Verification items for the finished model (mm, model axes). A direction names the side the tool comes from. Round coordinates to 2 decimals unless told otherwise and drop trailing zeros. Write each loop counter-clockwise with the first axis right and the second up, starting at its lowest first coordinate (ties: lowest second). Pieces come first, ordered by that corner, then holes. Notation, with made-up numbers: (31, 43) - (74, 43) arc R16 ccw to (74, 58) - close; hole circle Ø8 at (6, 34). An arc over 180 degrees is marked (long way). Answer as a JSON object with one key per item and string values. Group by question number.
1) Section check B-B (y = -5.5). Enter the section's corners in (x, z).
2) Mould release check, pull along Z, two halves, no side actions. Record for faces 4 (the flat face through (165, 13, 7)), 5 (the flat face through (74, 13, 0)), 6 (the cylindrical face through (31.952, -14.132, 7.934)): +Z half, -Z half, draft (parallel to the pull), parting line (faces both ways), or undercut.
3) Section check C-C (y = 21.5). Enter the section's corners in (x, z).
4) Go/stop test with flat-tipped pins: pin 1 Ø20.5 at (x, y) = (0, 0) entering from -Z; pin 2 Ø3.5 at (x, z) = (135, 7.5) entering from +Y; pin 3 Ø3 at (x, z) = (30, 7.5) entering from -Y; pin 4 Ø5 at (x, z) = (0, 7.5) entering from -Y. Record where each tip stops, or that it passes through.
5) Set-up check for faces 1 (the cylindrical face through (42.446, 40.103, 7.24)), 2 (the cylindrical face through (118.314, -14.132, 6.425)), 3 (the cylindrical face through (55.4, 22.53, 7.4)): record each of +Z, -Z, +X, -X, +Y, -Y from which the full face is reachable in a straight line by a thin tool's end or side.
6) Section check A-A (x = 120). Enter the section's corners in (y, z), then the cut area to 3 significant figures.
7) Thickness scan on line 1 (X direction, y = 26, z = 4); line 2 (X direction, y = 41.25, z = 7.5); line 3 (Z direction, x = 75, y = 41). Record the ranges inside material, lowest first.
8) Section check D-D (x = 150). Enter the section's corners in (y, z).
Autodesk Inventor part; units mm, degrees
ref_plane "YZ Plane" through (0, 0, 0) normal (1, 0, 0) x (0, 1, 0)
ref_plane "XZ Plane" through (0, 0, 0) normal (0, 1, 0) x (-1, 0, 0)
ref_plane "XY Plane" through (0, 0, 0) normal (0, 0, 1) x (1, 0, 0)
sketch "Skizze1" plane through (0, 0, 0) normal (0, 0, 1) x (1, 0, 0)
  circle A0 centre (0, 0) radius 11.5
  circle A1 centre (15, 25.9808) radius 11.5
  circle A2 centre (30, 0) radius 11.5
  circle A3 centre (44.4291, 25.9808) radius 11.5
  circle A4 centre (60, 0) radius 11.5
  circle A5 centre (75, 25.9615) radius 11.5
  circle A6 centre (90, -0.0192) radius 11.5
  circle A7 centre (104.4291, 25.9615) radius 11.5
  circle A8 centre (120, 0) radius 11.5
  circle A9 centre (135, 25.9615) radius 11.5
  circle A10 centre (150, -0.0192) radius 11.5
  line L0 (-15, 42.9808) -> (165, 42.9808)
  line L1 (165, 42.9808) -> (165, -17.0192)
  line L2 (165, -17.0192) -> (-15, -17.0192)
  line L3 (-15, -17.0192) -> (-15, 42.9808)
  dimension "d0" = 23
  dimension "d2" = 23
  dimension "d3" = 30
  dimension "d4" = 23
  dimension "d7" = 30
  dimension "d8" = 30
  dimension "d9" = 23
  dimension "d10" = 29.4291
  dimension "d11" = 23
  dimension "d12" = 23
  dimension "d13" = 23
  dimension "d14" = 30
  dimension "d15" = 23
  dimension "d16" = 29.4291
  dimension "d24" = 23
  dimension "d25" = 23
  dimension "d26" = 23
  dimension "d27" = 30
  dimension "d28" = 15
  dimension "d31" = 15
  dimension "d36" = 180
  dimension "d98" = 60
  dimension "d99" = 5.5
  dimension "d100" = 52.4567
  dimension "d101" = 5.5192
  dimension "d102" = 5.5
  dimension "d103" = 5.5
extrude "Extrusion1" add sketch "Skizze1" along normal blind 15
hole "Bohrung1" at (120, -17.0192, 7.5) at (30, -17.0192, 7.5) at (0, -17.0192, 7.5) at (60, -17.0192, 7.5) at (150, -17.0192, 7.5) at (90, -17.0192, 7.5) direction (0, 1, 0) diameter 4 depth 8
thread "Gewinde2"
thread "Gewinde3"
sketch "Skizze4" plane through (-15, 42.9808, 0) normal (0, 1, 0) x (1, 0, 0)
  line L0 (180, 0) -> (180, -15)
  line L1 (150, 13) -> (150, -28.8024) construction
  line L2 (30, 13) -> (30, -28.8024) construction
  line L3 (119.4291, 13) -> (119.4291, -28.8024) construction
  line L4 (90, 13) -> (90, -28.8024) construction
  line L5 (59.4291, 13) -> (59.4291, -28.8024) construction
  line L6 (180, -15) -> (0, -15)
  line L7 (0, -15) -> (180, 0) construction
  line L8 (180, -15) -> (0, 0) construction
  line L9 (4.4998, -7.5) -> (175.5002, -7.5) construction
  point P0 (15, 0)
  point P1 (119.4291, -7.5)
  point P2 (150, -7.5)
  point P3 (90, -7.5)
  point P4 (59.4291, -7.5)
  point P5 (30, -7.5)
  point P6 (90, -7.5)
  point P7 (90, -7.5)
  dimension "d58" = 30
  dimension "d60" = 60.5709
  dimension "d62" = 90
  dimension "d64" = 120.5709
  dimension "d66" = 150
  dimension "d85" = 0
  dimension "d86" = 0
  dimension "d87" = 0
  dimension "d88" = 0
  dimension "d89" = 0
hole "Bohrung2" at (104.4291, 42.9808, 7.5) at (135, 42.9808, 7.5) at (75, 42.9808, 7.5) at (44.4291, 42.9808, 7.5) at (15, 42.9808, 7.5) direction (0, -1, 0) diameter 4 depth 8 tip angle 118
thread "Gewinde4"
thread "Gewinde5"
thread "Gewinde6"
thread "Gewinde7"
thread "Gewinde8"
properties part number "Ventilhalter" material "Aluminium 6061"
Returned:
{
 "1": {"outline": "(-15, 0) - (-10.1, 0) - (-10.1, 15) - (-15, 15) - close; (10.1, 0) - (19.9, 0) - (19.9, 15) - (10.1, 15) - close; (40.1, 0) - (49.9, 0) - (49.9, 15) - (40.1, 15) - close; (70.1, 0) - (79.89, 0) - (79.89, 15) - (70.1, 15) - close; (100.11, 0) - (109.9, 0) - (109.9, 15) - (100.11, 15) - close; (130.1, 0) - (139.89, 0) - (139.89, 15) - (130.1, 15) - close; (160.11, 0) - (165, 0) - (165, 15) - (160.11, 15) - close"},
 "2": {"face 4": "draft", "face 5": "-Z half", "face 6": "undercut"},
 "3": {"outline": "(-15, 0) - (4.41, 0) - (4.41, 15) - (-15, 15) - close; (25.59, 0) - (33.84, 0) - (33.84, 15) - (25.59, 15) - close; (55.02, 0) - (64.4, 0) - (64.4, 15) - (55.02, 15) - close; (85.6, 0) - (93.83, 0) - (93.83, 15) - (85.6, 15) - close; (115.03, 0) - (124.4, 0) - (124.4, 15) - (115.03, 15) - close; (145.6, 0) - (165, 0) - (165, 15) - (145.6, 15) - close"},
 "4": {"pin 1": "through", "pin 2": "y = 14.6", "pin 3": "y = 11.4", "pin 4": "y = -17.02"},
 "5": {"face 1": "+Y", "face 2": "-Y", "face 3": "+Z, -Z"},
 "6": {"outline": "(-17.02, 0) - (-11.5, 0) - (-11.5, 5.5) - (-17.02, 5.5) - close; (-17.02, 9.5) - (-11.5, 9.5) - (-11.5, 15) - (-17.02, 15) - close; (11.5, 0) - (42.98, 0) - (42.98, 15) - (11.5, 15) - close", "area": "533 mm2"},
 "7": {"line 1": "-15 to 3.5, 26.5 to 32.93, 55.93 to 63.5, 86.5 to 92.93, 115.93 to 123.5, 146.5 to 165", "line 2": "-15 to 13, 17 to 42.43, 46.43 to 73, 77 to 102.43, 106.43 to 133, 137 to 165", "line 3": "0 to 5.5, 9.5 to 15"},
 "8": {"outline": "(-17.02, 0) - (-11.52, 0) - (-11.52, 5.5) - (-17.02, 5.5) - close; (-17.02, 9.5) - (-11.52, 9.5) - (-11.52, 15) - (-17.02, 15) - close; (11.48, 0) - (42.98, 0) - (42.98, 15) - (11.48, 15) - close"}
}
